Can you work these out from the model? Positions are in its coordinate system, mm. A direction names the side the tool comes from. Give positions to 0.01 mm unless a question says otherwise; leave off trailing zeros. Loops run counter-clockwise (first coordinate to the right, second up) from the corner with the lowest first, then second, coordinate; pieces in that order, holes last. Notation, with made-up numbers: (28, 49.5) - (50, 49.5) arc R18 cw to (50, 58.5) - close; hole circle Ø7 at (70, -12). An arc over 180 degrees is marked (long way). Answer as a JSON object with one key per item and string values. Group by question number.
Item 1: Will these pins go through, and if not, where does the flat tip stop? pin 1 (6 mm diameter, centred on y = 21, z = 7.5, fed in from -X); pin 2 (3 mm diameter, centred on x = 5.4, z = -10.71, fed in from -Y); pin 3 (10 mm diameter, centred on y = 16, z = 6.5, fed in from +X); pin 4 (3 mm diameter, centred on x = -6, z = 10, fed in from -Y).
Item 2: Suppose I cut it at A-A on z = 0. Write out the boundary of the cut face in (x, y).
Item 3: Suppose I cut it at C-C on y = 18.5. Write out the boundary of the cut face in (x, z).
Item 4: Please list where these lines run through material, in increasing order: L1, parallel to X at y = 30.5, z = 0; L2, parallel to Y at x = 8, z = 1; L3, parallel to Z at x = 1.5, y = 42.5.
Item 5: Which directions (+Z, -Z, +X, -X, +Y, -Y) give clear straight access to the entire face, cutting with the end or side of a thin tool? Please do faces 1 (the flat face through (-3.4, 0, 3.4)), 2 (the flat face through (-7, 3.1, 9)).
Item 6: Thinking about a two-plate mould opening in X: for faces 3 (the cylindrical face through (4.699, 24.72, 6.128)), 4 (the flat face through (-3.43, 5, 7.09)), 5 (the flat face through (9, 3.1, 4)), which applies, pulls with the +X half, pulls with the -X half, needs draft (parallel to the pull), parting line crosses it, or undercut?
Item 7: Suppose I cut it at B-B on x = 0. Write out the boundary of the cut face in (y, z), and give its area (3 significant figures).
Item 8: Suppose I cut it at D-D on x = 13. Write out the boundary of the cut face in (y, z).
from build123d import *

# Parameters (mm, degrees)
SKETCH_1_R          = 16.47426238
SKETCH_1_R_2        = 1.75
SKETCH_1_R_3        = 7.722310491
EXTRUDE_1_DEPTH     = 5
SKETCH_1_3_R        = 7.722310491
SKETCH_1_3_R_2      = 4.118565595
EXTRUDE_2_DEPTH     = 45
SKETCH_2_R          = 3
CUT_EXTRUDE_1_DEPTH = 3.1


with BuildPart() as part:
    # Sketch 1 → Extrude 1 (new body)
    with BuildSketch(Plane(origin=(0, 0, 0), x_dir=(1, 0, 0), z_dir=(0, 1, 0))):
        with Locations(Location((0, 0, 0), (0, 0, 270))):
            Circle(SKETCH_1_R)
        with Locations(Location((10.714869681, -5.402922146, 0), (0, 0, 270))):
            Circle(SKETCH_1_R_2, mode=Mode.SUBTRACT)
        with Locations(Location((5.402922146, 10.714869681, 0), (0, 0, 270))):
            Circle(SKETCH_1_R_2, mode=Mode.SUBTRACT)
        with Locations(Location((-10.714869681, 5.402922146, 0), (0, 0, 270))):
            Circle(SKETCH_1_R_2, mode=Mode.SUBTRACT)
        with Locations(Location((-5.402922146, -10.714869681, 0), (0, 0, 270))):
            Circle(SKETCH_1_R_2, mode=Mode.SUBTRACT)
        with Locations(Location((0, 0, 0), (0, 0, 270))):
            Circle(SKETCH_1_R_3, mode=Mode.SUBTRACT)
    extrude(amount=EXTRUDE_1_DEPTH)

    # Sketch 1_3 → Extrude 2 (add)
    with BuildSketch(Plane(origin=(0, 0, 0), x_dir=(1, 0, 0), z_dir=(0, 1, 0))):
        with Locations(Location((0, 0, 0), (0, 0, 90))):
            Circle(SKETCH_1_3_R)
        with Locations(Location((0, 0, 0), (0, 0, 90))):
            Circle(SKETCH_1_3_R_2, mode=Mode.SUBTRACT)
    extrude(amount=EXTRUDE_2_DEPTH)

    # Sketch 2 → Cut-Extrude 1 (cut)
    with BuildSketch(Plane.XZ):
        with Locations(Location((5.402922146, -10.714869681, 0), (0, 0, 270))):
            Circle(SKETCH_2_R)
        with Locations(Location((-10.714869681, -5.402922146, 0), (0, 0, 270))):
            Circle(SKETCH_2_R)
        with Locations(Location((-5.402922146, 10.714869681, 0), (0, 0, 270))):
            Circle(SKETCH_2_R)
        with Locations(Location((10.714869681, 5.402922146, 0), (0, 0, 270))):
            Circle(SKETCH_2_R)
    extrude(amount=-CUT_EXTRUDE_1_DEPTH, mode=Mode.SUBTRACT)


solid = part.part
Worked out:
{
 "1": {"pin 1": "stops at x = -6.28", "pin 2": "passes through", "pin 3": "stops at x = 7.58", "pin 4": "stops at y = 3.1"},
 "2": {"outline": "(-16.47, 0) - (-4.12, 0) - (-4.12, 45) - (-7.72, 45) - (-7.72, 5) - (-16.47, 5) - close; (4.12, 0) - (16.47, 0) - (16.47, 5) - (7.72, 5) - (7.72, 45) - (4.12, 45) - close"},
 "3": {"outline": "circle Ø15.44 at (0, 0); hole circle Ø8.24 at (0, 0)"},
 "4": {"L1": "x = -7.72 to -4.12, 4.12 to 7.72", "L2": "y = 0 to 5", "L3": "z = -7.58 to -3.84, 3.84 to 7.58"},
 "5": {"face 1": "+Z, -Z, +X, -X, -Y", "face 2": "-Y"},
 "6": {"face 3": "parting line crosses it", "face 4": "needs draft", "face 5": "undercut"},
 "7": {"outline": "(0, -16.47) - (5, -16.47) - (5, -7.72) - (45, -7.72) - (45, -4.12) - (0, -4.12) - close; (0, 4.12) - (45, 4.12) - (45, 7.72) - (5, 7.72) - (5, 16.47) - (0, 16.47) - close", "area": "412 mm2"},
 "8": {"outline": "(0, -10.12) - (5, -10.12) - (5, 10.12) - (0, 10.12) - (0, 7.35) - (3.1, 7.35) - (3.1, 3.46) - (0, 3.46) - close"}
}
